```python
from build123d import *

# Parameters (mm, degrees)
SKETCH1_R           = 15
BOSS_EXTRUDE1_DEPTH = 4.5
SKETCH3_R           = 7
BOSS_EXTRUDE2_DEPTH = 10
SKETCH4_R           = 4
CUT_EXTRUDE1_DEPTH  = 15
SKETCH5_R           = 2
CUT_EXTRUDE2_DEPTH  = 10


with BuildPart() as part:
    # Sketch1 → Boss-Extrude1 (new body)
    with BuildSketch(Plane(origin=(0, 0, 0), x_dir=(1, 0, 0), z_dir=(0, 1, 0))):
        Circle(SKETCH1_R)
    extrude(amount=BOSS_EXTRUDE1_DEPTH)

    # Sketch3 → Boss-Extrude2 (add)
    with BuildSketch(Plane(origin=(0, 4.5, 0), x_dir=(1, 0, 0), z_dir=(0, 1, 0))):
        Circle(SKETCH3_R)
    extrude(amount=BOSS_EXTRUDE2_DEPTH)

    # Sketch4 → Cut-Extrude1 (cut)
    with BuildSketch(Plane(origin=(0, 14.5, 0), x_dir=(1, 0, 0), z_dir=(0, 1, 0))):
        Circle(SKETCH4_R)
    extrude(amount=-CUT_EXTRUDE1_DEPTH, mode=Mode.SUBTRACT)

    # Sketch5 → Cut-Extrude2 (cut)
    with BuildSketch(Plane(origin=(0, 4.5, 0), x_dir=(1, 0, 0), z_dir=(0, 1, 0))):
        with Locations((0, 12)):
            Circle(SKETCH5_R)
        with Locations((12, 0)):
            Circle(SKETCH5_R)
        with Locations((0, -12)):
            Circle(SKETCH5_R)
        with Locations((-12, 0)):
            Circle(SKETCH5_R)
    extrude(amount=-CUT_EXTRUDE2_DEPTH, mode=Mode.SUBTRACT)


solid = part.part
```
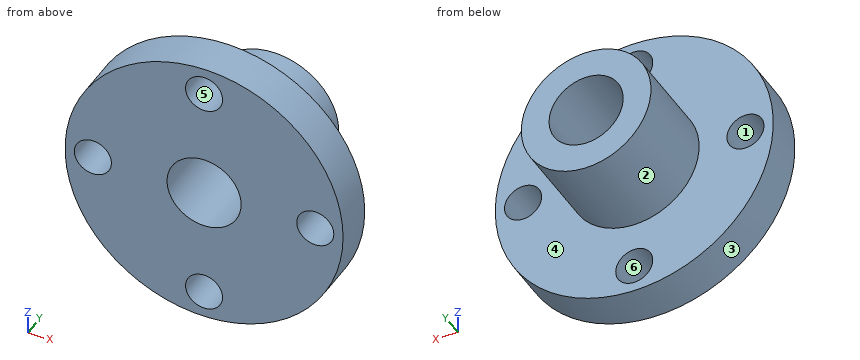
Input: part model. Units: mm. Frame: model coordinates. Face numbers are marked on the shaded views. A direction names the side the tool comes from. Coordinates: 2 decimals unless noted, no trailing zeros. Loops run counter-clockwise (first coordinate to the right, second up) from the corner with the lowest first, then second, coordinate; pieces in that order, holes last. Notation, with made-up numbers: (78, -18) -> (125, -18) arc R11 ccw to (125, -5) -> close; hole circle Ø1 at (-22, 41.25). An arc over 180 degrees is marked (long way). Use a Markdown table: item, result.
1) Material intervals for line 1 along Z through (x, y) = (0, 2.4); line 2 along X through (y, z) = (11.5, 0), sorted ascending. Write a range as from..to.
Results found:
| item | result |
|---|---|
| line 1 | z = -15..-14, -10..-4, 4..10, 14..15 |
| line 2 | x = -7..-4, 4..7 |
2) Cut plane D-D (x = -12). Return the cut outline in (y, z).
Results found:
| item | result |
|---|---|
| outline | (0, -9) -> (4.5, -9) -> (4.5, -2) -> (0, -2) -> close; (0, 2) -> (4.5, 2) -> (4.5, 9) -> (0, 9) -> close |
3) Cut plane C-C (z = 0). Return the cut outline in (x, y).
Results found:
| item | result |
|---|---|
| outline | (-15, 0) -> (-14, 0) -> (-14, 4.5) -> (-15, 4.5) -> close; (-10, 0) -> (-4, 0) -> (-4, 14.5) -> (-7, 14.5) -> (-7, 4.5) -> (-10, 4.5) -> close; (4, 0) -> (10, 0) -> (10, 4.5) -> (7, 4.5) -> (7, 14.5) -> (4, 14.5) -> close; (14, 0) -> (15, 0) -> (15, 4.5) -> (14, 4.5) -> close |
4) Access query for the marked faces 1 and 2. Directions: +Z, -Z, +X, -X, +Y, -Y. A direction counts if a zero-diameter tool reaches every point of the face in a straight line with its end or side. Return the directions, or none.
Results found:
| item | result |
|---|---|
| face 1 | +Y, -Y |
| face 2 | +Y |
5) Cut plane B-B (x = 0). Return the cut outline in (y, z).
Results found:
| item | result |
|---|---|
| outline | (0, -15) -> (4.5, -15) -> (4.5, -14) -> (0, -14) -> close; (0, -10) -> (4.5, -10) -> (4.5, -7) -> (14.5, -7) -> (14.5, -4) -> (0, -4) -> close; (0, 4) -> (14.5, 4) -> (14.5, 7) -> (4.5, 7) -> (4.5, 10) -> (0, 10) -> close; (0, 14) -> (4.5, 14) -> (4.5, 15) -> (0, 15) -> close |
6) Pull-direction query (Z, two-part tool) for the marked faces 3, 4, 5 and 6; classes: released by +Z, released by -Z, zero draft, split by the parting line, or undercut.
Results found:
| item | result |
|---|---|
| face 3 | split by the parting line |
| face 4 | zero draft |
| face 5 | undercut |
| face 6 | undercut |
7) Contact query for flat-ended pins moving along their axis: pin 1 (4 mm diameter, centred on y = 2.5, z = -3.5, fed in from -X); pin 2 (4 mm diameter, centred on x = -10, y = 4.5, fed in from -Z). Output: stop coordinate, or through.
Results found:
| item | result |
|---|---|
| pin 1 | stops at x = -14.92 |
| pin 2 | stops at z = -12.69 |
8) Cut plane A-A (z = -12). Return the cut outline in (x, y).
Results found:
| item | result |
|---|---|
| outline | (-9, 0) -> (-2, 0) -> (-2, 4.5) -> (-9, 4.5) -> close; (2, 0) -> (9, 0) -> (9, 4.5) -> (2, 4.5) -> close |
